Check sheet for the modelled part. Datum: model origin and axes. Units: mm. A direction names the side the tool comes from. Round coordinates to 2 decimals unless told otherwise and drop trailing zeros. Order: outer loops, then holes, each group sorted by start corner. A loop starts at its lowest first (then second) coordinate and runs counter-clockwise, first axis right, second up. Notation, with made-up numbers: (38, 80) -> (83, 80) arc R29 ccw to (83, 118) -> close; hole circle Ø7 at (-29.75, 48.25). An arc over 180 degrees is marked (long way). Use CSV: the item, a comma, the result in double quotes.
```python
from build123d import *

# Parameters (mm, degrees)
DODANIE_WYCI_GNI_CIE1_DEPTH = 8
SZKIC2_R                    = 0.478785513
WYTNIJ_WYCI_GNI_CIE1_DEPTH  = 0.1
SZKIC3_R                    = 0.5
WYTNIJ_WYCI_GNI_CIE2_DEPTH  = 0.1


with BuildPart() as part:
    # Szkic1 → Dodanie-wyciągnięcie1 (new body)
    with BuildSketch(Plane.XY):
        with BuildLine():
            Line((-56.651560295, 21.778571429), (-56.851560295, 21.778571429))
            Line((-56.851560295, 21.778571429), (-56.851560295, -3.421428571))
            ThreePointArc((-56.851560295, -3.421428571), (-56.265773857, -4.835642134), (-54.851560295, -5.421428571))
            Line((-54.851560295, -5.421428571), (-39.851560295, -5.421428571))
            ThreePointArc((-39.851560295, -5.421428571), (-38.437346732, -4.835642134), (-37.851560295, -3.421428571))
            Line((-37.851560295, -3.421428571), (-37.851560295, 21.778571429))
            Line((-37.851560295, 21.778571429), (-38.051560295, 21.778571429))
            Line((-38.051560295, 21.778571429), (-38.051560295, -3.221428571))
            ThreePointArc((-38.051560295, -3.221428571), (-38.637346732, -4.635642134), (-40.051560295, -5.221428571))
            Line((-40.051560295, -5.221428571), (-54.651560295, -5.221428571))
            ThreePointArc((-54.651560295, -5.221428571), (-56.065773857, -4.635642134), (-56.651560295, -3.221428571))
            Line((-56.651560295, -3.221428571), (-56.651560295, 21.778571429))
        make_face()
    extrude(amount=DODANIE_WYCI_GNI_CIE1_DEPTH)

    # Szkic2 → Wytnij-wyciągnięcie1 (cut)
    with BuildSketch(Plane(origin=(-37.851560295, 0, 0), x_dir=(0, 0, -1), z_dir=(1, 0, 0))):
        with Locations((-6, 15.528571429)):
            Circle(SZKIC2_R)
        with Locations((-2, 15.528571429)):
            Circle(SZKIC2_R)
        with Locations((-2, 2.828571429)):
            Circle(SZKIC2_R)
        with Locations((-6, 2.828571429)):
            Circle(SZKIC2_R)
    extrude(amount=-WYTNIJ_WYCI_GNI_CIE1_DEPTH, mode=Mode.SUBTRACT)

    # Szkic3 → Wytnij-wyciągnięcie2 (cut)
    with BuildSketch(Plane.ZY.offset(56.851560295)):
        with Locations((6, 15.528571429)):
            Circle(SZKIC3_R)
        with Locations((2, 15.528571429)):
            Circle(SZKIC3_R)
        with Locations((2, 2.828571429)):
            Circle(SZKIC3_R)
        with Locations((6, 2.828571429)):
            Circle(SZKIC3_R)
    extrude(amount=-WYTNIJ_WYCI_GNI_CIE2_DEPTH, mode=Mode.SUBTRACT)


solid = part.part
```
Q1. Go/stop test with flat-tipped pins: pin 1 (3 mm diameter, centred on x = -54, z = 5, fed in from +Y); pin 2 (1.1 mm diameter, centred on y = 15.5, z = 6, fed in from -X); pin 3 (0.8 mm diameter, centred on y = 15.5, z = 2, fed in from +X); pin 4 (6 mm diameter, centred on x = -51.5, y = 14.5, fed in from -Z). Record where each tip stops, or that it passes through.
Result sheet:
pin 1,"stops at y = -5.03"
pin 2,"stops at x = -56.85"
pin 3,"stops at x = -37.95"
pin 4,"passes through"
Q2. Sectioned sample at A-A, the plane y = 0.25. Enter the section's corners in (x, z).
Result sheet:
outline,"(-56.85, 0) -> (-56.65, 0) -> (-56.65, 8) -> (-56.85, 8) -> close; (-38.05, 0) -> (-37.85, 0) -> (-37.85, 8) -> (-38.05, 8) -> close"
Q3. Sectioned sample at B-B, the plane z = 2. Enter the section's corners in (x, y).
Result sheet:
outline,"(-56.85, -3.42) arc R2 ccw to (-54.85, -5.42) -> (-39.85, -5.42) arc R2 ccw to (-37.85, -3.42) -> (-37.85, 2.35) -> (-37.95, 2.35) -> (-37.95, 3.31) -> (-37.85, 3.31) -> (-37.85, 15.05) -> (-37.95, 15.05) -> (-37.95, 16.01) -> (-37.85, 16.01) -> (-37.85, 21.78) -> (-38.05, 21.78) -> (-38.05, -3.22) arc R2 cw to (-40.05, -5.22) -> (-54.65, -5.22) arc R2 cw to (-56.65, -3.22) -> (-56.65, 21.78) -> (-56.85, 21.78) -> (-56.85, 16.03) -> (-56.75, 16.03) -> (-56.75, 15.03) -> (-56.85, 15.03) -> (-56.85, 3.33) -> (-56.75, 3.33) -> (-56.75, 2.33) -> (-56.85, 2.33) -> close"
Q4. Sectioned sample at C-C, the plane x = -46.5. Enter the section's corners in (y, z), then the cut area to 3 significant figures.
Result sheet:
outline,"(-5.42, 0) -> (-5.22, 0) -> (-5.22, 8) -> (-5.42, 8) -> close"
area,"1.60 mm^2"
Q5. Scan lines: L1, parallel to X at y = 5, z = 0.75; L2, parallel to Y at x = -43.75, z = 3.25; L3, parallel to Y at x = -39.5, z = 0.5. Record each from-to range of solid material in increasing order.
Result sheet:
L1,"x = -56.85 to -56.65, -38.05 to -37.85"
L2,"y = -5.42 to -5.22"
L3,"y = -5.39 to -5.14"
Q6. Access from +Z, -Z, +X, -X, +Y, -Y to the whole of each face (thin tool, end or side, straight path). Record for faces 1 (the face through (-56.652, 9, 4)), 2 (the face through (-56.852, 9, 4)).
Result sheet:
face 1,"+Z, -Z, +Y"
face 2,"+Z, -Z, -X, +Y, -Y"
